```python
from build123d import *

# Parameters (mm, degrees)
SKETCH_2_OUTSIDE_W  = 53.464
SKETCH_2_OUTSIDE_H  = 53.464
CUT_EXTRUDE_1_DEPTH = 20
CHAMFER_1_SIZE      = 1
SKETCH_3_R          = 3
CUT_EXTRUDE_2_DEPTH = 3
CUT_EXTRUDE_2_DRAFT = -40


with BuildPart() as part:
    # Эскиз1 → Повернуть1 (revolve)
    with BuildSketch(Plane(origin=(0, 0, 0), x_dir=(1, 0, 0), z_dir=(0, 1, 0)), mode=Mode.PRIVATE) as revolve_1_sk:
        Polygon((-64.645142278, 0), (-64.645142278, 8), (-60.645142278, 8), (-60.645142278, 6), (59.354857722, 6), (59.354857722, 11), (79.354857722, 11), (79.354857722, 0), align=None)
    revolve(revolve_1_sk.sketch.rotate(Axis((-81.575248185, 0, 0), (1, 0, 0)), 180), axis=Axis((-81.575248185, 0, 0), (1, 0, 0)))

    # Эскиз2 outside → Вырез-Вытянуть1 (cut)
    with BuildSketch(Plane(origin=(79.354857722, 0, 0), x_dir=(0, 0, -1), z_dir=(1, 0, 0))):
        Rectangle(SKETCH_2_OUTSIDE_W, SKETCH_2_OUTSIDE_H)
        Polygon((10.969655115, 0), (5.484827557, 9.5), (-5.484827557, 9.5), (-10.969655115, 0), (-5.484827557, -9.5), (5.484827557, -9.5), align=None, mode=Mode.SUBTRACT)
    extrude(amount=-CUT_EXTRUDE_1_DEPTH, mode=Mode.SUBTRACT)

    # Фаска1
    chamfer_1_edges = [part.edges().sort_by_distance(p)[0] for p in [
        (79.354857722, -4.75, -8.227241336),
        (79.354857722, -9.5, 0),
        (79.354857722, -4.75, 8.227241336),
        (79.354857722, 4.75, 8.227241336),
        (79.354857722, 9.5, 0),
        (79.354857722, 4.75, -8.227241336),
    ]]
    chamfer(chamfer_1_edges, length=CHAMFER_1_SIZE)


with BuildPart() as cut_extrude_2_tool:
    # Эскиз3 → Вырез-Вытянуть2 (with draft: the straight prism first)
    with BuildSketch(Plane.ZY.offset(64.645142278)):
        Circle(SKETCH_3_R)
    extrude(amount=-CUT_EXTRUDE_2_DEPTH)
    # Вырез-Вытянуть2: the draft: its side faces are tilted about the plane it starts from
    cut_extrude_2_sides = [cut_extrude_2_tool.faces().sort_by_distance(p)[0] for p in [
        (-63.145142278, 0, -3),
    ]]
    draft(cut_extrude_2_sides, Plane.ZY.offset(64.645142278), CUT_EXTRUDE_2_DRAFT)


with BuildPart() as part_1:
    add(part.part)

    # Вырез-Вытянуть2: cut by cut_extrude_2_tool
    add(cut_extrude_2_tool.part, mode=Mode.SUBTRACT)


solid = part_1.part
```
Work out the finished part from the listing and answer in its coordinate system (mm). A direction names the side the tool comes from. Round coordinates to 2 decimals unless told otherwise and drop trailing zeros. Return JSON: item names as keys, results as strings. Group by question number.
Q1. Each of these flat-tipped pins is pushed along its axis until it touches: pin 1 Ø8 at (x, z) = (-30, -1.5) entering from +Y; pin 2 Ø0.8 at (y, z) = (0, 0) entering from -X; pin 3 Ø6 at (x, z) = (-3.5, 3.5) entering from -Y; pin 4 Ø3 at (y, z) = (-6, -7.5) entering from +X. Where does it stop, or does it pass through?
Q2. The mould has two halves that part along X. Classify faces 4 (the cylindrical face through (0.195, -1.802, 5.723)), 5 (the flat face through (69, 9.5, 0)), 6 (the flat face through (79.355, 0, 0)), 7 (the flat face through (59.355, -4, -5)): released by +X, released by -X, zero draft, split by the parting line, or undercut.
Q3. For faces 1 (the flat face through (-60.645, -6, -2)), 2 (the flat face through (68.988, 4.684, -8.266)), 3 (the cylindrical face through (-62.62, 7.81, -1.73)), determine the directions among +Z, -Z, +X, -X, +Y, -Y from which every point of the face is accessible in a straight line to the end or side of a thin tool.
Q4. Find the intervals of material crossed by L1, parallel to X at y = 6.5, z = 4.5; L2, parallel to Z at x = 24, y = 0.25; L3, parallel to X at y = -8.5, z = -3.75, in increasing order.
Solved:
{
 "1": {"pin 1": "y = 6", "pin 2": "x = -61.65", "pin 3": "y = -5.98", "pin 4": "x = 79.35"},
 "2": {"face 4": "undercut", "face 5": "zero draft", "face 6": "released by +X", "face 7": "undercut"},
 "3": {"face 1": "none", "face 2": "-Z, +X, -X, +Y", "face 3": "-X"},
 "4": {"L1": "-64.65 to -60.65, 59.35 to 79.35", "L2": "-5.99 to 5.99", "L3": "59.35 to 79.35"}
}
